Read the model definition and answer for the solid it produces. Units are mm, in the model's axes. A direction names the side the tool comes from. Coordinates: 2 decimals unless noted, no trailing zeros. Write each loop counter-clockwise with the first axis right and the second up, starting at its lowest first coordinate (ties: lowest second). Pieces come first, ordered by that corner, then holes. Notation, with made-up numbers: (-39, 20) - (-28, 20) arc R21 cw to (-28, 55) - close; hole circle Ø1 at (-3.5, 23.25). An arc over 180 degrees is marked (long way). Use a Markdown table: item, result.
from build123d import *

# Parameters (mm, degrees)
EXTRUDE_THIN1_START = -7.9375
EXTRUDE_THIN1_DEPTH = 15.875
SKETCH4_R           = 2.3495
EXTRUDE3_DEPTH      = 67.428185443


# Read off the part's stored shape, not the designer's step: Extrude-Thin1
with BuildPart() as part:
    # Extrude-Thin1 outline → Extrude-Thin1 (new body)
    with BuildSketch(Plane(origin=(0, 0, 0), x_dir=(1, 0, 0), z_dir=(0, 1, 0)).offset(EXTRUDE_THIN1_START)):
        with BuildLine():
            Line((3.79480894, -1.778), (50.8, -1.778))
            Line((50.8, -1.778), (50.8, 0))
            Line((50.8, 0), (3.79480894, 0))
            ThreePointArc((3.79480894, 0), (1.6127938, -1.133475), (1.285491529, -3.57044625))
            Line((1.285491529, -3.57044625), (17.2085, -47.79652213))
            Line((17.2085, -47.79652213), (18.881378275, -47.19422463))
            Line((18.881378275, -47.19422463), (2.958369803, -2.96814875))
            ThreePointArc((2.958369803, -2.96814875), (3.06747056, -2.155825), (3.79480894, -1.778))
        make_face()
    extrude(amount=EXTRUDE_THIN1_DEPTH)

    # Sketch4 → Extrude3 (cut, through all)
    with BuildSketch(Plane(origin=(3.556, 0, 1.778), x_dir=(1, 0, 0), z_dir=(0, 0, 1))):
        with Locations((38.354, 0)):
            Circle(SKETCH4_R)
        with Locations((15.24, 0)):
            Circle(SKETCH4_R)
    extrude(amount=-EXTRUDE3_DEPTH, mode=Mode.SUBTRACT)

    # Cut-Extrude1 cone 1 section (through the dimple's axis) → Cut-Extrude1 (revolve, cut)
    with BuildSketch(Plane(origin=(41.91, 0, 1.778), x_dir=(0, -1, 0), z_dir=(1, 0, 0))):
        Polygon((0, 0), (3.5433, 0), (0, 3.080143698), align=None)
    revolve(axis=Axis((41.91, 0, 1.778), (0, 0, -1)), mode=Mode.SUBTRACT)

    # Cut-Extrude1 cone 2 section (through the dimple's axis) → Cut-Extrude1 cone 2 (revolve, cut)
    with BuildSketch(Plane(origin=(18.796, 0, 1.778), x_dir=(0, -1, 0), z_dir=(1, 0, 0))):
        Polygon((0, 0), (3.5433, 0), (0, 3.080143698), align=None)
    revolve(axis=Axis((18.796, 0, 1.778), (0, 0, -1)), mode=Mode.SUBTRACT)


solid = part.part
(1) Each of these flat-tipped pins is pushed along its axis until it touches: P1, Ø1, axis at y = 0.5, z = 5.5, coming from the +X side; P2, Ø1, axis at y = -4.5, z = 30, coming from the -X side; P3, Ø1.5, axis at y = -5, z = 25.5, coming from the +X side. Where does it stop, or does it pass through?
Report:
| item | result |
|---|---|
| P1 | stops at x = 4.05 |
| P2 | stops at x = 10.62 |
| P3 | stops at x = 11.34 |
(2) Straight lines are drawn through the part: L1, parallel to X at y = 0, z = 0.4; L2, parallel to Y at x = 41.91, z = 0.6; L3, parallel to Z at x = 22, y = 7. For each, find the intervals that lie inside material, in ascending order.
Report:
| item | result |
|---|---|
| L1 | x = 2.39 to 16.45, 21.15 to 39.56, 44.26 to 50.8 |
| L2 | y = -7.94 to -2.35, 2.35 to 7.94 |
| L3 | z = 0 to 1.78 |
(3) A cutting plane is placed at A-A, the plane y = 0. Write down the section's boundary in (x, z).
Report:
| item | result |
|---|---|
| outline | (1.29, 3.57) arc R2.67 ccw to (3.79, 0) - (16.45, 0) - (16.45, 0.74) - (15.25, 1.78) - (3.79, 1.78) arc R0.89 cw to (2.96, 2.97) - (18.88, 47.19) - (17.21, 47.8) - close; (21.15, 0) - (39.56, 0) - (39.56, 0.74) - (38.37, 1.78) - (22.34, 1.78) - (21.15, 0.74) - close; (44.26, 0) - (50.8, 0) - (50.8, 1.78) - (45.45, 1.78) - (44.26, 0.74) - close |
(4) A cutting plane is placed at C-C, the plane y = -5.25. Write down the section's boundary in (x, z).
Report:
| item | result |
|---|---|
| outline | (1.29, 3.57) arc R2.67 ccw to (3.79, 0) - (50.8, 0) - (50.8, 1.78) - (3.79, 1.78) arc R0.89 cw to (2.96, 2.97) - (18.88, 47.19) - (17.21, 47.8) - close |
(5) For faces 4 (the flat face through (11.03, -0.11, 25.39)), 5 (the cylindrical face through (1.634, -0.111, 1.104)), 6 (the cylindrical face through (21.037, 0.706, 0.375)), determine the directions among +Z, -Z, +X, -X, +Y, -Y from which every point of the face is accessible in a straight line to the end or side of a thin tool.
Report:
| item | result |
|---|---|
| face 4 | +X, +Y, -Y |
| face 5 | -X, +Y, -Y |
| face 6 | -Z |
(6) The mould has two halves that part along Z. Classify faces 1 (the cylindrical face through (3.06, -0.11, 2.17)), 2 (the flat face through (7, -7.938, 17)), 3 (the flat face through (9, 0, 25)): pulls with the +Z half, pulls with the -Z half, needs draft (parallel to the pull), parting line crosses it, or undercut.
Report:
| item | result |
|---|---|
| face 1 | undercut |
| face 2 | needs draft |
| face 3 | pulls with the +Z half |
(7) A cutting plane is placed at B-B, the plane x = 41.91. Write down the section's boundary in (y, z).
Report:
| item | result |
|---|---|
| outline | (-7.94, 0) - (-2.35, 0) - (-2.35, 0.74) - (-3.54, 1.78) - (-7.94, 1.78) - close; (2.35, 0) - (7.94, 0) - (7.94, 1.78) - (3.54, 1.78) - (2.35, 0.74) - close |
(8) A cutting plane is placed at D-D, the plane x = 7. Write down the section's boundary in (y, z), and give its area (3 significant figures).
Report:
| item | result |
|---|---|
| outline | (-7.94, 0) - (7.94, 0) - (7.94, 1.78) - (-7.94, 1.78) - close; (-7.94, 14.19) - (7.94, 14.19) - (7.94, 19.44) - (-7.94, 19.44) - close |
| area | 112 mm² |
